Geometry: final body of the model. Coordinates: model frame, mm. A direction names the side the tool comes from. Coordinates: 2 decimals unless noted, no trailing zeros. Order: outer loops, then holes, each group sorted by start corner. A loop starts at its lowest first (then second) coordinate and runs counter-clockwise, first axis right, second up. Notation, with made-up numbers: (19, 12.25) - (53, 12.25) arc R23 cw to (53, 32.25) - close; hole circle Ø4 at (-7, 2.5). An arc over 180 degrees is marked (long way). Use a Markdown table: item, result. Add a question column.
```python
from build123d import *

# Parameters (mm, degrees)
PAD_DEPTH       = 16
POCKET_DEPTH    = 7
SKETCH002_R     = 3.5
POCKET001_DEPTH = 42.001
SKETCH003_R     = 3.5
POCKET002_DEPTH = 7


with BuildPart() as part:
    # Sketch → Pad (new body)
    with BuildSketch(Plane.XZ):
        Polygon((-27.5, 7), (-27.5, 0), (-6.5, 0), (-6.5, 10), (6.5, 10), (6.5, 0), (27.5, 0), (27.5, 7), (14.5, 7), (14.5, 32), (4.5, 32), (4.5, 17), (-4.5, 17), (-4.5, 32), (-14.5, 32), (-14.5, 7), align=None)
    extrude(amount=PAD_DEPTH)

    # Sketch001 (on Face6 of Pad) → Pocket (cut)
    with BuildSketch(Plane(origin=(0, 0, 0), x_dir=(1, 0, 0), z_dir=(0, 0, -1))):
        Polygon((-27.5, 16), (-27.5, 10), (-20, 16), align=None)
        Polygon((20, 16), (27.5, 16), (27.5, 10), align=None)
    extrude(amount=-POCKET_DEPTH, mode=Mode.SUBTRACT)

    # Sketch002 (on Face12 of Pocket) → Pocket001 (cut, through all)
    with BuildSketch(Plane(origin=(14.5, 0, 0), x_dir=(0, 0, 1), z_dir=(1, 0, 0))):
        with Locations((24.5, 8)):
            Circle(SKETCH002_R)
    extrude(amount=-POCKET001_DEPTH, mode=Mode.SUBTRACT)

    # Sketch003 (on Face11 of Pocket001) → Pocket002 (cut)
    with BuildSketch(Plane(origin=(0, 0, 7), x_dir=(-1, 0, 0), z_dir=(0, 0, 1))):
        with Locations((21, 7)):
            Circle(SKETCH003_R)
        with Locations((-21, 7)):
            Circle(SKETCH003_R)
    extrude(amount=-POCKET002_DEPTH, mode=Mode.SUBTRACT)


solid = part.part
```
1) Section C-C (z = 5). Return loops of the section in (x, y).
2) Ray query, line 1 along X through (y, z) = (-7, 3); line 2 along X through (y, z) = (-2, 6); line 3 along X through (y, z) = (-12.5, 19). Return the intervals inside material, ascending.
3) Section D-D (y = -8). Give the number of separate pieces and of enclosed holes in the cut face, then the cut area to 3 significant figures.
4) Section A-A (x = -21). Return loops of the section in (y, z).
5) Set-up query: faces 1 (the face through (-6.5, -8, 5)), 2 (the face through (14.5, -8, 19)), 3 (the face through (-4.5, -4, 24)), 4 (the face through (9.57, -4.895, 26.115)), 5 (the face through (-18, -10, 7)). Return all of +Z, -Z, +X, -X, +Y, -Y with unobstructed straight access to the full face (end or side cutting, diameter ignored); none if empty.
6) Draft query along Y for faces 6 (the face through (0, -8, 10)), 7 (the face through (19.385, -3.895, 3.549)), 8 (the face through (0, -16, 16)). Return one class per face: pulls with the +Y half, pulls with the -Y half, needs draft (parallel to the pull), parting line crosses it, or undercut.
7) Section B-B (z = 30.5). Return loops of the section in (x, y).
8) Pin query (flat end, axial travel): pin 1 (2.5 mm diameter, centred on x = 0, y = -10.5, fed in from +Z); pin 2 (9 mm diameter, centred on y = -8, z = 24.5, fed in from -X); pin 3 (2 mm diameter, centred on x = 21, y = -13.5, fed in from +Z); pin 4 (4 mm diameter, centred on y = -8, z = 24.5, fed in from +X). Return the tip coordinate at first contact, or that it passes through.
Values follow:
| question | item | result |
|---|---|---|
| 1 | outline | (-27.5, -10) - (-20, -16) - (-6.5, -16) - (-6.5, 0) - (-27.5, 0) - close; (6.5, -16) - (20, -16) - (27.5, -10) - (27.5, 0) - (6.5, 0) - close; hole circle Ø7 at (-21, -7); hole circle Ø7 at (21, -7) |
| 2 | line 1 | x = -27.5 to -24.5, -17.5 to -6.5, 6.5 to 17.5, 24.5 to 27.5 |
| 2 | line 2 | x = -27.5 to -6.5, 6.5 to 27.5 |
| 2 | line 3 | x = -14.5 to -4.5, 4.5 to 14.5 |
| 3 | separate pieces | 5 |
| 3 | enclosed holes | 0 |
| 3 | area | 611 mm² |
| 4 | outline | (-15.2, 0) - (-10.5, 0) - (-10.5, 7) - (-15.2, 7) - close; (-3.5, 0) - (0, 0) - (0, 7) - (-3.5, 7) - close |
| 5 | face 1 | -Z, +Y, -Y |
| 5 | face 2 | +Z, +X, +Y, -Y |
| 5 | face 3 | +Z, +Y, -Y |
| 5 | face 4 | +X, -X |
| 5 | face 5 | +Z, -X, +Y, -Y |
| 6 | face 6 | needs draft |
| 6 | face 7 | undercut |
| 6 | face 8 | pulls with the -Y half |
| 7 | outline | (-14.5, -16) - (-4.5, -16) - (-4.5, 0) - (-14.5, 0) - close; (4.5, -16) - (14.5, -16) - (14.5, 0) - (4.5, 0) - close |
| 8 | pin 1 | stops at z = 17 |
| 8 | pin 2 | stops at x = -14.5 |
| 8 | pin 3 | stops at z = 7 |
| 8 | pin 4 | passes through |
